Geometry: final body of the model. Coordinates: model frame, mm. A direction names the side the tool comes from. Round coordinates to 2 decimals unless told otherwise and drop trailing zeros. Write each loop counter-clockwise with the first axis right and the second up, starting at its lowest first coordinate (ties: lowest second). Pieces come first, ordered by that corner, then holes. Notation, with made-up numbers: M -7,4 L 2,4 A35 ccw 2,43 Z; hole C 26.5,-36.75 d7. An arc over 180 degrees is marked long. Use one line per item in the form item = value. Start each with the question number.
Item 1: Section query A-A (z = -2.5). Return loops of the section in (x, y).
Item 2: Section query D-D (x = -1.5). Return loops of the section in (y, z).
Item 3: Pin query (flat end, axial travel): pin 1 Ø2.5 at (y, z) = (-24.75, -15.5) entering from +X; pin 2 Ø5 at (x, z) = (1.5, 2) entering from -Y; pin 3 Ø2 at (y, z) = (-25, -5.5) entering from -X. Return the tip coordinate at first contact, or that it passes through.
Item 4: Pull-direction query (Y, two-part tool) for faces 4 (the cylindrical face through (-8.6, 12.5, 2.2)), 5 (the cylindrical face through (-43.255, 26.287, -25.248)), 6 (the flat face through (2, -18.2, 2)); classes: pulls with the +Y half, pulls with the -Y half, needs draft (parallel to the pull), parting line crosses it, or undercut.
Item 5: Reachability of faces 1 (the cylindrical face through (10.4, -9.5, 2.2)), 2 (the flat face through (-42, 0, -21)), 3 (the cylindrical face through (-44.73, 23.43, -15.79)) from +Z, -Z, +X, -X, +Y, -Y: full face, straight path, thin tool, end or side. Return the list, or none.
Item 6: Ray query, probe 1 along Z at (x, y) = (-43.5, -20.5); probe 2 along Y at (x, z) = (-45.25, -15.5); probe 3 along Y at (x, z) = (-46, -6). Return the intervals inside material, ascending.
Item 7: Section query B-B (y = 7.5). Return loops of the section in (x, z), and give its area (3 significant figures).
Item 8: Section query C-C (x = 9.5). Return loops of the section in (y, z).
from build123d import *

# Parameters (mm, degrees)
SKETCH1_R           = 1.75
BOSS_EXTRUDE1_DEPTH = 4.5
SKETCH2_W           = 15
SKETCH2_H           = 54
BOSS_EXTRUDE2_DEPTH = 26
SKETCH5_W           = 21
SKETCH5_H           = 43
CUT_EXTRUDE1_DEPTH  = 15
SKETCH6_R           = 1.35
CUT_EXTRUDE2_DEPTH  = 12
CUT_EXTRUDE3_DEPTH  = 15
FILLET1_R           = 10
FILLET3_R           = 2.5


with BuildPart() as part:
    # Sketch1 → Boss-Extrude1 (new body)
    with BuildSketch(Plane.XY):
        Polygon((-13.65, -18.2), (13.65, -18.2), (13.65, 18.2), (-13.65, 18.2), (-23.65, 27), (-50.65, 27), (-50.65, -27), (-23.65, -27), align=None)
        with Locations((-9.5, 11)):
            Circle(SKETCH1_R, mode=Mode.SUBTRACT)
        with Locations(Location((9.5, 11, 0), (0, 0, 180))):
            Circle(SKETCH1_R, mode=Mode.SUBTRACT)
        with Locations(Location((-9.5, -11, 0), (0, 0, 180))):
            Circle(SKETCH1_R, mode=Mode.SUBTRACT)
        with Locations((9.5, -11)):
            Circle(SKETCH1_R, mode=Mode.SUBTRACT)
    extrude(amount=BOSS_EXTRUDE1_DEPTH)

    # Sketch2 → Boss-Extrude2 (add)
    with BuildSketch(Plane(origin=(0, 0, 0), x_dir=(-1, 0, 0), z_dir=(0, 0, -1))):
        with Locations((43.15, 0)):
            Rectangle(SKETCH2_W, SKETCH2_H)
    extrude(amount=BOSS_EXTRUDE2_DEPTH)

    # Sketch5 → Cut-Extrude1 (cut)
    with BuildSketch(Plane(origin=(-35.65, 0, 0), x_dir=(0, 0, -1), z_dir=(1, 0, 0))):
        with Locations((10.5, 0)):
            Rectangle(SKETCH5_W, SKETCH5_H)
    extrude(amount=-CUT_EXTRUDE1_DEPTH, mode=Mode.SUBTRACT)

    # Sketch6 → Cut-Extrude2 (cut)
    with BuildSketch(Plane.ZY.offset(50.65)):
        with Locations((-15.5, 24.75)):
            Circle(SKETCH6_R)
        with Locations(Location((-5.5, 24.75, 0), (0, 0, 180))):
            Circle(SKETCH6_R)
        with Locations((-5.5, -24.75)):
            Circle(SKETCH6_R)
        with Locations(Location((-15.5, -24.75, 0), (0, 0, 180))):
            Circle(SKETCH6_R)
    extrude(amount=-CUT_EXTRUDE2_DEPTH, mode=Mode.SUBTRACT)

    # Sketch8 → Cut-Extrude3 (cut)
    with BuildSketch(Plane.ZY.offset(50.65)):
        with BuildLine():
            Line((-15.5, -21.5), (-5.5, -21.5))
            ThreePointArc((-5.5, -21.5), (-10.5, -23.75), (-15.5, -21.5))
        make_face()
    extrude(amount=-CUT_EXTRUDE3_DEPTH, mode=Mode.SUBTRACT)

    # Fillet1
    fillet1_edges = [part.edges().sort_by_distance(p)[0] for p in [
        (-13.65, -18.2, 2.25),
        (-23.65, -27, 2.25),
        (-23.65, 27, 2.25),
        (-13.65, 18.2, 2.25),
    ]]
    fillet(fillet1_edges, radius=FILLET1_R)

    # Fillet3
    fillet3_edges = [part.edges().sort_by_distance(p)[0] for p in [
        (-43.15, 27, -26),
        (-43.15, -27, -26),
        (-50.65, 0, 0),
        (-50.65, 0, -21),
    ]]
    fillet(fillet3_edges, radius=FILLET3_R - 0.0001)  # a hair under: the kernel refuses the full size


solid = part.part
Working result:
q1.outline = M -50.65,-27 L -35.65,-27 L -35.65,-21.5 L -50.65,-21.5 Z; M -50.65,21.5 L -35.65,21.5 L -35.65,27 L -50.65,27 Z
q2.outline = M -18.2,0 L 18.2,0 L 18.2,4.5 L -18.2,4.5 Z
q3.pin_1 = -35.65
q3.pin_2 = -18.2
q3.pin_3 = -38.65
q4.face_4 = undercut
q4.face_5 = pulls with the +Y half
q4.face_6 = pulls with the -Y half
q5.face_1 = +Z, -Z
q5.face_2 = +X, -X
q5.face_3 = -X
q6.probe_1 = -26 to -21, 0 to 4.5
q6.probe_2 = -27 to -26.1, -23.4 to -21.5, 21.5 to 23.4, 26.1 to 27
q6.probe_3 = -27 to -26, -23.5 to -22.01, 21.5 to 23.5, 26 to 27
q7.outline = M -50.65,-26 L -35.65,-26 L -35.65,-21 L -48.15,-21 A2.5 ccw -50.65,-23.5 Z; M -50.65,2.5 A2.5 ccw -48.15,0 L 13.65,0 L 13.65,4.5 L -50.65,4.5 Z
q7.area = 362 mm²
q8.outline = M -18.2,0 L -12.75,0 L -12.75,4.5 L -18.2,4.5 Z; M -9.25,0 L 9.25,0 L 9.25,4.5 L -9.25,4.5 Z; M 12.75,0 L 18.2,0 L 18.2,4.5 L 12.75,4.5 Z
